Geometry check sheet. Reference: the model listing, model coordinates, mm. A direction names the side the tool comes from. Coordinates: 2 decimals unless noted, no trailing zeros. Write each loop counter-clockwise with the first axis right and the second up, starting at its lowest first coordinate (ties: lowest second). Pieces come first, ordered by that corner, then holes.
Autodesk Inventor part; units mm, degrees
ref_plane "YZ Plane" through (0, 0, 0) normal (1, 0, 0) x (0, 1, 0)
ref_plane "XZ Plane" through (0, 0, 0) normal (0, 1, 0) x (-1, 0, 0)
ref_plane "XY Plane" through (0, 0, 0) normal (0, 0, 1) x (1, 0, 0)
sketch "スケッチ1" plane through (0, 0, 0) normal (0, 0, 1) x (1, 0, 0)
  line L0 (-12.5, -12.5) -> (12.5, -12.5) construction
  line L1 (12.5, -12.5) -> (12.5, 12.5) construction
  line L2 (12.5, 12.5) -> (-12.5, 12.5) construction
  line L3 (-12.5, 12.5) -> (-12.5, -12.5) construction
  line L4 (-12.5, -12.5) -> (12.5, 12.5) construction
  line L5 (12.5, -12.5) -> (-12.5, 12.5) construction
  line L6 (-8.1, 12.5) -> (-12.5, 12.5)
  line L7 (-12.5, 12.5) -> (-12.5, 8.1)
  line L8 (8.1, 12.5) -> (12.5, 12.5)
  line L9 (12.5, 12.5) -> (12.5, 8.1)
  line L10 (-12.5, -8.1) -> (-12.5, -12.5)
  line L11 (-12.5, -12.5) -> (-8.1, -12.5)
  line L12 (8.1, -12.5) -> (12.5, -12.5)
  line L13 (12.5, -12.5) -> (12.5, -8.1)
  line L14 (-6, 12.5) -> (-6, 14.5)
  line L15 (-6, 14.5) -> (6, 14.5)
  line L16 (6, 14.5) -> (6, 12.5)
  arc A0 (-8.1, 12.5) -> (-6, 12.5) centre (-7.05, 12.5) ccw
  arc A1 (6, 12.5) -> (8.1, 12.5) centre (7.05, 12.5) ccw
  line L17 (0, 12.5) -> (0, 0) construction
  line L18 (0, 0) -> (12.5, 0) construction
  line L19 (-12.5, 6) -> (-14.5, 6) construction
  line L20 (-14.5, 6) -> (-14.5, -6) construction
  line L21 (-14.5, -6) -> (-12.5, -6) construction
  arc A2 (-12.5, 6) -> (-12.5, 8.1) centre (-12.5, 7.05) ccw
  arc A3 (-12.5, -8.1) -> (-12.5, -6) centre (-12.5, -7.05) ccw construction
  line L22 (-6, -12.5) -> (-6, -14.5)
  line L23 (-6, -14.5) -> (6, -14.5)
  line L24 (6, -14.5) -> (6, -12.5)
  arc A4 (-6, -12.5) -> (-8.1, -12.5) centre (-7.05, -12.5) ccw
  arc A5 (8.1, -12.5) -> (6, -12.5) centre (7.05, -12.5) ccw
  line L25 (12.5, 6) -> (14.5, 6) construction
  line L26 (14.5, 6) -> (14.5, -6) construction
  line L27 (14.5, -6) -> (12.5, -6) construction
  arc A6 (12.5, 8.1) -> (12.5, 6) centre (12.5, 7.05) ccw construction
  arc A7 (12.5, -6) -> (12.5, -8.1) centre (12.5, -7.05) ccw construction
  line L28 (-9.05, 12.5) -> (-5.95, 12.5) construction
  line L29 (-5.95, 12.5) -> (-5.95, 9.5) construction
  line L30 (-5.95, 9.5) -> (-9.05, 9.5) construction
  line L31 (-9.05, 9.5) -> (-9.05, 12.5) construction
  line L32 (-12.5, 9.05) -> (-9.5, 9.05) construction
  line L33 (-9.5, 5.95) -> (-12.5, 5.95) construction
  line L34 (-12.5, 5.95) -> (-12.5, 9.05) construction
  line L35 (-7.5, 12.5) -> (-7.5, 9.5) construction
  line L36 (-9.5, 7.5) -> (-12.5, 7.5) construction
  line L37 (-12.5, -12.5) -> (-12.5, 12.5)
  line L38 (12.5, -12.5) -> (12.5, 12.5)
  line L39 (0, -14.5) -> (0, 14.5) construction
  circle A8 centre (0, -8.5) radius 1.35
  circle A9 centre (8.5, 0) radius 1.35
  circle A10 centre (0, 8.5) radius 1.35
  circle A11 centre (-8.5, 0) radius 1.35
  circle A12 centre (0, 0) radius 5.01
  circle A13 centre (0, 0) radius 10.51
  point P0 (-12.5, 6)
  dimension "d0" = 25
  dimension "d1" = 1.05
  dimension "d2" = 2
  dimension "d3" = 6.5
  dimension "d4" = 3.1
  dimension "d6" = 3
  dimension "d17" = 5
  dimension "d18" = 5
  dimension "d46" = 25
  dimension "d58" = 2.7
  dimension "d59" = 8.5
  dimension "d62" = 360
  dimension "d64" = 10.02
  dimension "d65" = 21.02
extrude "押し出し1" add sketch "スケッチ1" along normal blind 5 contours A0 L14 L15 L16 A1 L8 L9 L38 L13 L12 A5 L24 L23 L22 A4 L11 L10 L37 A2 L7 L6
sketch "スケッチ2" plane through (-12.5, -12.5, 5) normal (0, -1, 0) x (1, 0, 0)
  line L0 (12.5, 0) -> (12.5, -5.2657) construction
  line L1 (0, -2.5) -> (22.3, -2.5) construction
  line L2 (0, -5) -> (0, 0)
  line L3 (6.5, 0) -> (18.5, 0)
  line L4 (25, -5) -> (25, 0)
  point P0 (12.5, -5)
  point P1 (2.7, -2.5)
  point P2 (0, -10)
  point P3 (25, -10)
  dimension "d55" = 2.5
  dimension "d56" = 2.7
  dimension "d57" = 2.7
hole "穴1" at (-9.8, -12.5, 2.5) at (9.8, -12.5, 2.5) direction (0, 1, 0) diameter 2.459 depth 8.8
pattern_circular "円形状パターン1" count 2 over 360 about axis through (0, 0, -10) along (0, 0, 1) of "穴1"
extrude "押し出し7" add sketch "スケッチ1" along normal blind 2.5 contours A13
equation "\"d18\" = d17"
equation "\"d57\" = d56"
properties part number "頭_サーボホーンフレーム" material "アセタール樹脂、黒"
1. Thickness scan on line 1 along X through (y, z) = (-11, 2.4); line 2 along Z through (x, y) = (9.8, 8.25); line 3 along X through (y, z) = (9.5, 3.5). Record the ranges inside material, lowest first.
Computed values:
line 1: x = -12.5 to -11.03, -8.57 to 8.57, 11.03 to 12.5
line 2: z = 0 to 1.27, 3.73 to 5
line 3: x = -12.5 to -10.52, -9.08 to -4.5, 4.5 to 9.08, 10.52 to 12.5
2. Access from +Z, -Z, +X, -X, +Y, -Y to the whole of each face (thin tool, end or side, straight path). Record for faces 4 (the flat face through (6, -14, 2)), 5 (the flat face through (-6, 13, 2)), 6 (the flat face through (2, -5, 2.5)), 7 (the flat face through (-6, -13, 2)), 8 (the flat face through (10, 3.7, 3)).
Computed values:
face 4: +Z, -Z, +X, -Y
face 5: +Z, -Z, -X, +Y
face 6: +Z
face 7: +Z, -Z, -X, -Y
face 8: +Y
3. Gauge pin test, flat ends, axial feed: pin 1 Ø0.6 at (y, z) = (14, 3) entering from -X; pin 2 Ø1.3 at (x, z) = (10, 3.5) entering from +Y; pin 3 Ø2.5 at (x, y) = (8.5, 0) entering from +Z; pin 4 Ø0.6 at (y, z) = (-13, 2) entering from +X. Record the tip position at first contact, or that the pin passes through.
Computed values:
pin 1: stops at x = -6
pin 2: stops at y = 12.5
pin 3: passes through
pin 4: stops at x = 6
4. Sectioned sample at B-B, the plane z = 4.55. Record the boundary of the cut face in (x, y).
Computed values:
outline: (-12.5, -12.5) - (-8.1, -12.5) arc R1.05 cw to (-6, -12.5) - (-6, -14.5) - (6, -14.5) - (6, -12.5) arc R1.05 cw to (8.1, -12.5) - (12.5, -12.5) - (12.5, 12.5) - (8.1, 12.5) arc R1.05 cw to (6, 12.5) - (6, 14.5) - (-6, 14.5) - (-6, 12.5) arc R1.05 cw to (-8.1, 12.5) - (-12.5, 12.5) - (-12.5, 8.1) arc R1.05 cw to (-12.5, 6) - close; hole circle Ø21.02 at (0, 0)
5. Sectioned sample at C-C, the plane x = 7.5. Record the boundary of the cut face in (y, z), and give its area (3 significant figures).
Computed values:
outline: (-11.55, 0) - (-0.91, 0) - (-0.91, 2.5) - (-7.36, 2.5) - (-7.36, 5) - (-11.55, 5) - close; (0.91, 0) - (11.55, 0) - (11.55, 5) - (7.36, 5) - (7.36, 2.5) - (0.91, 2.5) - close
area: 74.2 mm2
6. Sectioned sample at A-A, the plane y = 0. Record the boundary of the cut face in (x, z), and give its area (3 significant figures).
Computed values:
outline: (-12.5, 0) - (-9.85, 0) - (-9.85, 2.5) - (-10.51, 2.5) - (-10.51, 5) - (-12.5, 5) - close; (-7.15, 0) - (-5.01, 0) - (-5.01, 2.5) - (-7.15, 2.5) - close; (5.01, 0) - (7.15, 0) - (7.15, 2.5) - (5.01, 2.5) - close; (9.85, 0) - (12.5, 0) - (12.5, 5) - (10.51, 5) - (10.51, 2.5) - (9.85, 2.5) - close
area: 33.9 mm2
7. Sectioned sample at D-D, the plane z = 0.5. Record the boundary of the cut face in (x, y), and give its area (3 significant figures).
Computed values:
outline: (-12.5, -12.5) - (-8.1, -12.5) arc R1.05 cw to (-6, -12.5) - (-6, -14.5) - (6, -14.5) - (6, -12.5) arc R1.05 cw to (8.1, -12.5) - (12.5, -12.5) - (12.5, 12.5) - (8.1, 12.5) arc R1.05 cw to (6, 12.5) - (6, 14.5) - (-6, 14.5) - (-6, 12.5) arc R1.05 cw to (-8.1, 12.5) - (-12.5, 12.5) - (-12.5, 8.1) arc R1.05 cw to (-12.5, 6) - close; hole circle Ø2.7 at (-8.5, 0); hole circle Ø10.02 at (0, 0); hole circle Ø2.7 at (0, -8.5); hole circle Ø2.7 at (0, 8.5); hole circle Ø2.7 at (8.5, 0)
area: 563 mm2
8. Draft check along Z on faces 1 (the flat face through (-9, 7, 5)), 2 (the flat face through (-11.3, -12.5, 2.5)), 3 (the cylindrical face through (-9.426, 4.648, 1.877)). Enter one of: released by +Z, released by -Z, zero draft, split by the parting line, or undercut.
Computed values:
face 1: released by +Z
face 2: zero draft
face 3: undercut
